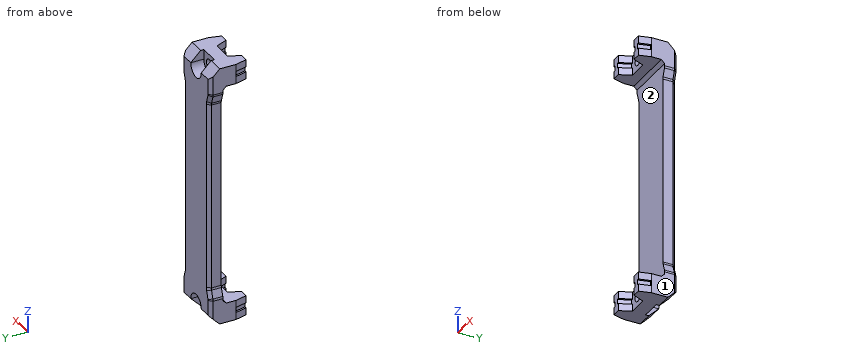
from build123d import *
from build123d.topology import SkipClean

# Parameters (mm, degrees)
EXTRUDE_1_DEPTH     = 4
EXTRUDE_3_DEPTH     = 6
CHAMFER_1_SIZE      = 3
CUT_EXTRUDE_2_DEPTH = 3.99
CUT_EXTRUDE_3_REACH = 51.222
SKETCH_7_R          = 1.5
SKETCH_8_R          = 6
EXTRUDE_4_DEPTH     = 1
FILLET_1_R          = 0.5
SKETCH_9_R          = 5
CUT_EXTRUDE_4_DEPTH = 3
SKETCH_10_R         = 3.55
CUT_EXTRUDE_5_DEPTH = 3.6
CUT_EXTRUDE_6_DEPTH = 0.8
CUT_EXTRUDE_7_DEPTH = 50.986598204
FILLET_2_R          = 2
CHAMFER_2_SIZE      = 1


with BuildPart() as part:
    # ｽｹｯﾁ1 → ﾎﾞｽ - 押し出し1 (new body)
    with BuildSketch(Plane(origin=(0, 0, 0), x_dir=(1, 0, 0), z_dir=(0, 1, 0))):
        with BuildLine():
            Line((-7.9, 0), (-7.9, -48))
            Line((-7.9, -48), (7.9, -48))
            Line((7.9, -48), (7.9, 0))
            ThreePointArc((7.9, 0), (0, 7.9), (-7.9, 0))
        make_face()
    extrude(amount=EXTRUDE_1_DEPTH)

    # ｽｹｯﾁ4 → ﾎﾞｽ - 押し出し3 (add)
    with BuildSketch(Plane.XY.offset(48)):
        Polygon((-7, -7.5), (-4.5, -7.5), (-3, -4), (3, -4), (4.5, -7.5), (7, -7.5), (7.9, -4), (7.9, 0), (-7.9, 0), (-7.9, -4), align=None)
    extrude(amount=-EXTRUDE_3_DEPTH)

    # 面取り1
    chamfer_1_edges = [part.edges().sort_by_distance(p)[0] for p in [
        (0, 4, 48),
    ]]
    chamfer(chamfer_1_edges, length=CHAMFER_1_SIZE)

    # ｽｹｯﾁ6 → ｶｯﾄ - 押し出し2 (cut)
    with BuildSketch(Plane(origin=(0, 4, 0), x_dir=(1, 0, 0), z_dir=(0, 1, 0))):
        with BuildLine():
            Line((-3, -45), (-3, -49))
            Line((-3, -49), (3, -49))
            Line((3, -49), (3, -45))
            ThreePointArc((3, -45), (0, -42), (-3, -45))
        make_face()
    extrude(amount=-CUT_EXTRUDE_2_DEPTH, mode=Mode.SUBTRACT)

    # ｽｹｯﾁ7 → ｶｯﾄ - 押し出し3 (cut, up to next)
    with BuildSketch(Plane(origin=(0, 0.01, 0), x_dir=(1, 0, 0), z_dir=(0, 1, 0)), mode=Mode.PRIVATE) as cut_extrude_3_sk1:
        with Locations(Location((0, -45, 0), (0, 0, 270))):
            Circle(SKETCH_7_R)
    cut_extrude_3_tool1 = extrude(cut_extrude_3_sk1.sketch, amount=-CUT_EXTRUDE_3_REACH, mode=Mode.PRIVATE) & part.part
    add(cut_extrude_3_tool1.solids().sort_by_distance((0, 0.01, 45))[0], mode=Mode.SUBTRACT)

    # ｽｹｯﾁ8 → ﾎﾞｽ - 押し出し4 (add)
    with BuildSketch(Plane.XZ):
        with Locations(Location((0, 0, 0), (0, 0, 90))):
            Circle(SKETCH_8_R)
    extrude(amount=EXTRUDE_4_DEPTH)

    # ﾌｨﾚｯﾄ1
    fillet_1_edges = [part.edges().sort_by_distance(p)[0] for p in [
        (0, 0, -6),
    ]]
    fillet(fillet_1_edges, radius=FILLET_1_R)

    # ｽｹｯﾁ9 → ｶｯﾄ - 押し出し4 (cut)
    with BuildSketch(Plane(origin=(0, 4, 0), x_dir=(1, 0, 0), z_dir=(0, 1, 0))):
        with Locations(Location((0, 0, 0), (0, 0, 270))):
            Circle(SKETCH_9_R)
    extrude(amount=-CUT_EXTRUDE_4_DEPTH, mode=Mode.SUBTRACT)

    # ｽｹｯﾁ10 → ｶｯﾄ - 押し出し5 (cut)
    with BuildSketch(Plane(origin=(0, 1, 0), x_dir=(1, 0, 0), z_dir=(0, 1, 0))):
        with Locations(Location((0, 0, 0), (0, 0, 270))):
            Circle(SKETCH_10_R)
    extrude(amount=-CUT_EXTRUDE_5_DEPTH, mode=Mode.SUBTRACT)

    # ｽｹｯﾁ11 → ｶｯﾄ - 押し出し6 (cut, symmetric)
    with BuildSketch(Plane.XY.offset(45)):
        Polygon((3, -4), (4.5, -7.5), (5.1, -7.5), (3.6, -4), align=None)
        Polygon((6.4, -7.5), (7, -7.5), (7.9, -4), (7.3, -4), align=None)
    cut_extrude_6 = extrude(amount=CUT_EXTRUDE_6_DEPTH, both=True, mode=Mode.SUBTRACT)

    # ﾐﾗｰ1: ｶｯﾄ - 押し出し6 across plane
    add(cut_extrude_6.mirror(Plane(origin=(0, 0, 0), x_dir=(0, 0, 1), z_dir=(1, 0, 0))), mode=Mode.SUBTRACT)

    # ｽｹｯﾁ12 → ｶｯﾄ - 押し出し7 (cut, through all)
    with SkipClean():  # the faces are left unmerged after this step: merging them gives an invalid solid
        with BuildSketch(Plane(origin=(0, 4, 0), x_dir=(1, 0, 0), z_dir=(0, 1, 0))):
            with BuildLine():
                Line((-7.9, 0), (-7.9, -40))
                Line((-7.9, -40), (-6.9, -37))
                Line((-6.9, -37), (-6.9, -3.847076812))
                ThreePointArc((-6.9, -3.847076812), (-7.645913941, -1.987460691), (-7.9, 0))
            make_face()
        cut_extrude_7 = extrude(amount=-CUT_EXTRUDE_7_DEPTH, mode=Mode.SUBTRACT)

    # ﾐﾗｰ2: ｶｯﾄ - 押し出し7 across plane
    with SkipClean():  # the faces are left unmerged after this step: merging them gives an invalid solid
        add(cut_extrude_7.mirror(Plane(origin=(0, 0, 0), x_dir=(0, 0, 1), z_dir=(1, 0, 0))), mode=Mode.SUBTRACT)

    # ﾌｨﾚｯﾄ2
    fillet_2_edges = [part.edges().sort_by_distance(p)[0] for p in [
        (-6.9, 2, 3.847076812),
        (-6.9, 2, 37),
        (-7.9, 2, 40),
        (6.9, 2, 3.847076812),
        (7.9, 2, 40),
        (6.9, 2, 37),
    ]]
    fillet(fillet_2_edges, radius=FILLET_2_R)

    # 面取り2
    chamfer_2_edges = [part.edges().sort_by_distance(p)[0] for p in [
        (-7.9, 4, 42.66227766),
        (0, 4, -7.9),
        (7.9, 4, 42.66227766),
        (0, 0, 42),
        (-7.874174915, 4, 40.004190834),
        (-7.4, 4, 38.5),
        (-6.925825085, 4, 36.995809166),
        (-6.9, 4, 20.505670679),
        (-6.951159371, 4, 3.886430103),
        (6.951159371, 4, 3.886430103),
        (6.9, 4, 20.505670679),
        (6.925825085, 4, 36.995809166),
        (7.4, 4, 38.5),
        (7.874174915, 4, 40.004190834),
    ]]
    chamfer(chamfer_2_edges, length=CHAMFER_2_SIZE)

    # Surface Cut 1
    split(bisect_by=Plane.XY.offset(8), keep=Keep.TOP)

    # ﾐﾗｰ4: part across plane


with BuildPart() as part_1:
    add(part.part)
    add(part.part.mirror(Plane.XY.offset(8)))


solid = part_1.part
Read the model definition and answer for the solid it produces. Units are mm, in the model's axes. Face numbers are marked on the shaded views. Round coordinates to 2 decimals unless told otherwise and drop trailing zeros. Write each loop counter-clockwise with the first axis right and the second up, starting at its lowest first coordinate (ties: lowest second). Pieces come first, ordered by that corner, then holes. Notation, with made-up numbers: (-2.5, 8) - (45.5, 8) arc R28 ccw to (45.5, 46) - close; hole circle Ø4 at (-8.75, -27.75). An arc over 180 degrees is marked (long way). Use a Markdown table: item, result.
(1) The part is cut by section A-A (y = -1.75). Write down the section's boundary in (x, z).
Reported:
| item | result |
|---|---|
| outline | (-7.9, -32) - (7.9, -32) - (7.9, -26) - (-7.9, -26) - close; (-7.9, 42) - (7.9, 42) - (7.9, 48) - (-7.9, 48) - close; hole circle Ø3 at (0, -29); hole circle Ø3 at (0, 45) |
(2) The part is cut by section B-B (x = 0). Write down the section's boundary in (y, z), then the cut area to 3 significant figures.
Reported:
| item | result |
|---|---|
| outline | (-4, -32) - (0.01, -32) - (0.01, -30.5) - (-4, -30.5) - close; (-4, -27.5) - (0.01, -27.5) - (0.01, -26) - (4, -26) - (4, 42) - (0.01, 42) - (0.01, 43.5) - (-4, 43.5) - (-4, 42) - (-1, 42) - (0, 41) - (0, -25) - (-1, -26) - (-4, -26) - close; (-4, 46.5) - (0.01, 46.5) - (0.01, 48) - (-4, 48) - close |
| area | 297 mm2 |
(3) The mould has two halves that part along Z. Classify the marked faces 1 and 2: released by +Z, released by -Z, zero draft, split by the parting line, or undercut.
Reported:
| item | result |
|---|---|
| face 1 | zero draft |
| face 2 | undercut |
(4) The part is cut by section D-D (z = 1). Write down the section's boundary in (x, y).
Reported:
| item | result |
|---|---|
| outline | (-6.9, 0) - (6.9, 0) - (6.9, 3) - (5.9, 4) - (-5.9, 4) - (-6.9, 3) - close |
(5) Each of these flat-tipped pins is pushed along its axis until it touches: pin 1 Ø8 at (x, z) = (-2, 7) entering from -Y; pin 2 Ø3 at (y, z) = (-0.5, 25.5) entering from +X; pin 3 Ø3.5 at (x, z) = (0, -29) entering from -Y. Where does it stop, or does it pass through?
Reported:
| item | result |
|---|---|
| pin 1 | y = 0 |
| pin 2 | x = 6.9 |
| pin 3 | y = -4 |
(6) The part is cut by section C-C (y = 1.75). Write down the section's boundary in (x, z).
Reported:
| item | result |
|---|---|
| outline | (-7.9, -31.25) - (-3, -31.25) - (-3, -29) arc R3 cw to (3, -29) - (3, -31.25) - (7.9, -31.25) - (7.9, -24.32) arc R2 ccw to (7.8, -23.69) - (7, -21.31) arc R2 cw to (6.9, -20.68) - (6.9, 36.68) arc R2 cw to (7, 37.31) - (7.8, 39.69) arc R2 ccw to (7.9, 40.32) - (7.9, 47.25) - (3, 47.25) - (3, 45) arc R3 cw to (-3, 45) - (-3, 47.25) - (-7.9, 47.25) - (-7.9, 40.32) arc R2 ccw to (-7.8, 39.69) - (-7, 37.31) arc R2 cw to (-6.9, 36.68) - (-6.9, -20.68) arc R2 cw to (-7, -21.31) - (-7.8, -23.69) arc R2 ccw to (-7.9, -24.32) - close |
(7) Straight lines are drawn through the part: line 1 along X through (y, z) = (-2.6, -29); line 2 along Z through (x, y) = (2.25, -2.25); line 3 along Y through (x, z) = (0.5, -0.5). For each, find the intervals that lie inside material, in ascending order. Write a range as [from, to].
Reported:
| item | result |
|---|---|
| line 1 | [-7.9, -1.5], [1.5, 7.9] |
| line 2 | [-32, -26], [42, 48] |
| line 3 | [0, 4] |
